The figure shows three views and two pictorial views of one solid part (mm, origin at its lowest corner). Answer the questions. A direction names the side the tool comes from. Give positions to 0.01 mm unless a question says otherwise; leave off trailing zeros. Loops run counter-clockwise (first coordinate to the right, second up) from the corner with the lowest first, then second, coordinate; pieces in that order, holes last. Notation, with made-up numbers: M -28.5,-21.75 L 13.5,-21.75 A20 ccw 13.5,4.25 Z; hole C 21,67.5 d2. An arc over 180 degrees is marked long. Answer in a Markdown table with one row per item. Add a question column.
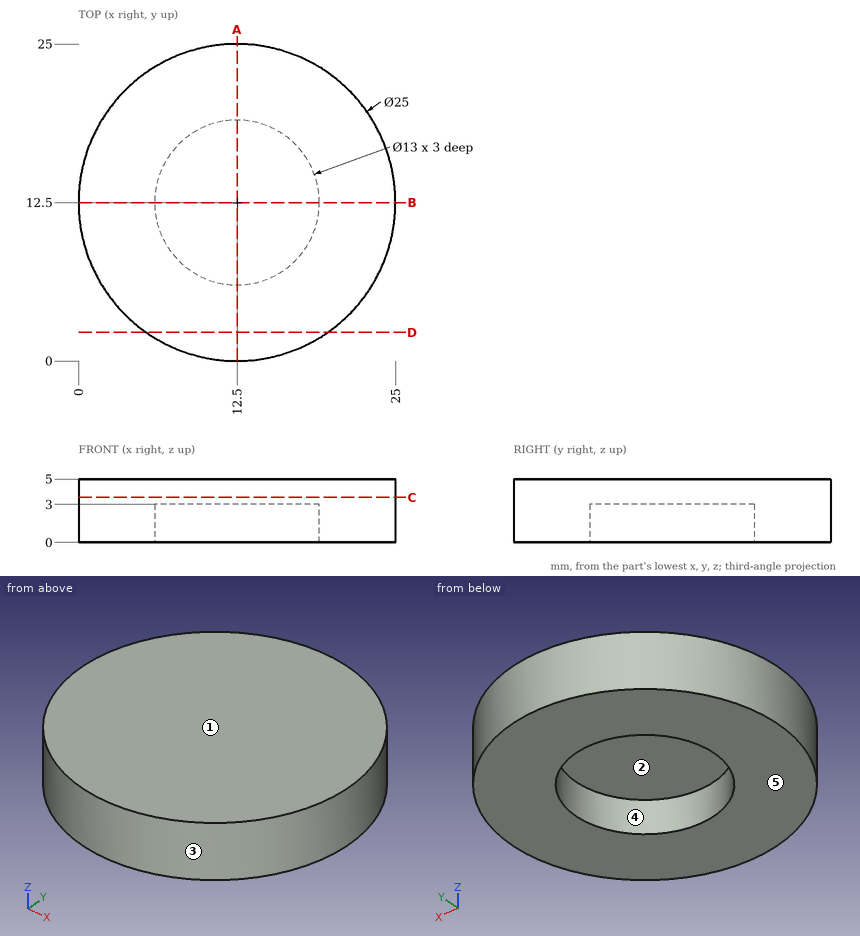
(1) Section A-A, the plane x = 12.5 is taken. Determine the outline of the cut face in (y, z), and give its area (3 significant figures).
(2) Consider line 1 along Y through (x, z) = (12.5, 1.1); line 2 along Y through (x, z) = (12.5, 3.6); line 3 along Z through (x, y) = (15.25, 13.25). Determine where each line is inside the solid, lowest interval first. Write a range as from..to.
(3) Section D-D, the plane y = 2.25 is taken. Determine the outline of the cut face in (x, z), and give its area (3 significant figures).
(4) Each of these flat-tipped pins is pushed along its axis until it touches: P1, Ø15, axis at x = 12.5, y = 12.5, coming from the -Z side; P2, Ø1.5, axis at x = 14.5, z = 2, coming from the +Y side; P3, Ø1.5, axis at x = 15.5, z = 3, coming from the +Y side; P4, Ø1, axis at x = 20.5, z = 2, coming from the -Y side. Where does it stop, or does it pass through?
(5) The mould has two halves that part along X. Classify the marked faces 1, 2 and 3: pulls with the +X half, pulls with the -X half, needs draft (parallel to the pull), parting line crosses it, or undercut.
(6) Section C-C, the plane z = 3.55 is taken. Determine the outline of the cut face in (x, y), and give its area (3 significant figures).
(7) Which of the six approach directions +Z, -Z, +X, -X, +Y, -Y give full straight-line access (tool end or side, diameter ignored) to the marked faces 4 and 5?
Numbers:
| question | item | result |
|---|---|---|
| 1 | outline | M 0,0 L 6,0 L 6,3 L 19,3 L 19,0 L 25,0 L 25,5 L 0,5 Z |
| 1 | area | 86.0 mm² |
| 2 | line 1 | y = 0..6, 19..25 |
| 2 | line 2 | y = 0..25 |
| 2 | line 3 | z = 3..5 |
| 3 | outline | M 5.35,0 L 19.65,0 L 19.65,5 L 5.35,5 Z |
| 3 | area | 71.5 mm² |
| 4 | P1 | stops at z = 0 |
| 4 | P2 | stops at y = 24.94 |
| 4 | P3 | stops at y = 24.8 |
| 4 | P4 | stops at y = 2.5 |
| 5 | face 1 | needs draft |
| 5 | face 2 | undercut |
| 5 | face 3 | parting line crosses it |
| 6 | outline | C 12.5,12.5 d25 |
| 6 | area | 491 mm² |
| 7 | face 4 | -Z |
| 7 | face 5 | -Z, +X, -X, +Y, -Y |
